Build history of the part. All positions in model axes, mm. A direction names the side the tool comes from. Give positions to 0.01 mm unless a question says otherwise; leave off trailing zeros. Order: outer loops, then holes, each group sorted by start corner. A loop starts at its lowest first (then second) coordinate and runs counter-clockwise, first axis right, second up. Notation, with made-up numbers: (8.5, -14.75) - (49.5, -14.75) arc R25 cw to (49.5, 7.25) - close; hole circle Ø9 at (60.25, -11.75). An arc over 180 degrees is marked (long way). Answer in a Markdown table with one row per item.
```python
from build123d import *

# Parameters (mm, degrees)
SKETCH1_R           = 9.5
BOSS_EXTRUDE1_DEPTH = 35
EXTRUDE_THIN1_START = 0.5
SKETCH1_4_R         = 5.5
SKETCH1_4_R_2       = 5
EXTRUDE_THIN1_DEPTH = 28.5
BOSS_EXTRUDE2_START = 0.8
SKETCH1_5_R         = 8.5
SKETCH1_5_R_2       = 5
BOSS_EXTRUDE2_DEPTH = 28
BOSS_EXTRUDE3_START = 0.3
SKETCH1_6_R         = 9.5
SKETCH1_6_R_2       = 8.5
BOSS_EXTRUDE3_DEPTH = 30
BOSS_EXTRUDE4_START = 1
BOSS_EXTRUDE4_DEPTH = 1
FILLET1_R           = 0.5
SKETCH4_R           = 2.15
CUT_EXTRUDE3_DEPTH  = 48.968739894
CHAMFER1_SIZE       = 1


with BuildPart() as part:
    # Sketch1 → Boss-Extrude1 (new body)
    with BuildSketch(Plane(origin=(0, 0, 0), x_dir=(0, 0, -1), z_dir=(1, 0, 0))):
        Polygon((-20, -5), (-18.5, -3.5), (-18.5, 8), (-9.5, 8), (-5, 13), (5, 13), (9.5, 8), (18.5, 8), (18.5, -3.5), (20, -5), (20, -13), (10, -13), (8.5, -11.5), (-8.5, -11.5), (-10, -13), (-20, -13), align=None)
        Circle(SKETCH1_R, mode=Mode.SUBTRACT)
    extrude(amount=BOSS_EXTRUDE1_DEPTH)



with BuildPart() as body_2:
    # Sketch1_4 → Extrude-Thin1 (new body)
    with BuildSketch(Plane(origin=(0, 0, 0), x_dir=(0, 0, -1), z_dir=(1, 0, 0)).offset(EXTRUDE_THIN1_START)):
        Circle(SKETCH1_4_R)
        Circle(SKETCH1_4_R_2, mode=Mode.SUBTRACT)
    extrude(amount=EXTRUDE_THIN1_DEPTH)

    # Sketch1_5 → Boss-Extrude2 (add)
    with BuildSketch(Plane(origin=(0, 0, 0), x_dir=(0, 0, -1), z_dir=(1, 0, 0)).offset(BOSS_EXTRUDE2_START)):
        Circle(SKETCH1_5_R)
        with Locations(Location((0, 0, 0), (0, 0, 180))):
            Circle(SKETCH1_5_R_2, mode=Mode.SUBTRACT)
    extrude(amount=BOSS_EXTRUDE2_DEPTH)


with BuildPart() as part_1:
    add(part.part)

    add(body_2.part)  # Boss-Extrude3 merges body 2
    # Sketch1_6 → Boss-Extrude3 (add)
    with BuildSketch(Plane(origin=(0, 0, 0), x_dir=(0, 0, -1), z_dir=(1, 0, 0)).offset(BOSS_EXTRUDE3_START)):
        Circle(SKETCH1_6_R)
        Circle(SKETCH1_6_R_2, mode=Mode.SUBTRACT)
    extrude(amount=BOSS_EXTRUDE3_DEPTH)

    # Sketch3 → Boss-Extrude4 (add)
    with BuildSketch(Plane(origin=(30.3, 0, 0), x_dir=(0, 0, -1), z_dir=(1, 0, 0)).offset(BOSS_EXTRUDE4_START)):
        with BuildLine():
            Line((-1.015917942, -8.43907049), (-1.1354377, -9.431902312))
            ThreePointArc((-1.1354377, -9.431902312), (0, 9.5), (1.1354377, -9.431902312))
            Line((1.1354377, -9.431902312), (1.015917942, -8.43907049))
            ThreePointArc((1.015917942, -8.43907049), (1.500925976, -7.394796464), (2.647576922, -7.499355735))
            ThreePointArc((2.647576922, -7.499355735), (4.216931478, -7.125074609), (3.386935643, -5.741576507))
            ThreePointArc((3.386935643, -5.741576507), (0, 6.666110848), (-3.386935643, -5.741576507))
            ThreePointArc((-3.386935643, -5.741576507), (-4.216931478, -7.125074609), (-2.647576922, -7.499355735))
            ThreePointArc((-2.647576922, -7.499355735), (-1.500925976, -7.394796464), (-1.015917942, -8.43907049))
        make_face()
    extrude(amount=BOSS_EXTRUDE4_DEPTH)

    # Fillet1
    fillet1_edges = [part_1.edges().sort_by_distance(p)[0] for p in [
        (35, -4.25, 19.25),
        (35, -9, 20),
        (0, 2.25, 18.5),
        (0, 8, 14),
        (0, 10.5, 7.25),
        (0, 13, 0),
        (0, 10.5, -7.25),
        (0, 8, -14),
        (0, 2.25, -18.5),
        (0, -4.25, -19.25),
        (0, -9, -20),
        (0, -9, 20),
        (0, -4.25, 19.25),
        (17.5, -3.5, 18.5),
        (17.5, 8, 18.5),
        (17.5, 8, 9.5),
        (17.5, 13, 5),
        (17.5, 13, -5),
        (17.5, 8, -9.5),
        (17.5, 8, -18.5),
        (17.5, -3.5, -18.5),
        (17.5, -5, -20),
        (17.5, -5, 20),
        (35, -9, -20),
        (35, -4.25, -19.25),
        (35, 2.25, -18.5),
        (35, 8, -14),
        (35, 10.5, -7.25),
        (35, 13, 0),
        (35, 10.5, 7.25),
        (35, 8, 14),
        (35, 2.25, 18.5),
    ]]
    fillet(fillet1_edges, radius=FILLET1_R)

    # Sketch4 → Cut-Extrude3 (cut, through all)
    with BuildSketch(Plane.XZ.offset(13)):
        with Locations(Location((7, 14, 0), (0, 0, 270))):
            Circle(SKETCH4_R)
        with Locations(Location((28, 14, 0), (0, 0, 270))):
            Circle(SKETCH4_R)
        with Locations(Location((28, -14, 0), (0, 0, 270))):
            Circle(SKETCH4_R)
        with Locations(Location((7, -14, 0), (0, 0, 270))):
            Circle(SKETCH4_R)
    extrude(amount=-CUT_EXTRUDE3_DEPTH, mode=Mode.SUBTRACT)

    # Chamfer1
    chamfer1_edges = [part_1.edges().sort_by_distance(p)[0] for p in [
        (7, 8, -11.85),
        (28, 8, -11.85),
        (28, 8, 16.15),
        (28, -13, 16.15),
        (7, 8, 16.15),
        (7, -13, 16.15),
    ]]
    chamfer(chamfer1_edges, length=CHAMFER1_SIZE)


solid = part_1.part
```
1. Drop flat-ended pins along their axis: P1, Ø2, axis at x = 20, z = 15.5, coming from the +Y side; P2, Ø9.5, axis at y = 2.5, z = -1.5, coming from the +X side; P3, Ø4, axis at x = 7, z = 13, coming from the +Y side. Give the stop position or say it passes through.
Check result:
| item | result |
|---|---|
| P1 | stops at y = 8 |
| P2 | stops at x = 32.3 |
| P3 | stops at y = 7.85 |
2. Cut at A-A on z = -14. Write the cut outline in (x, y).
Check result:
| item | result |
|---|---|
| outline | (0, -13) - (4.85, -13) - (4.85, 7) - (3.85, 8) - (0.5, 8) arc R0.5 ccw to (0, 7.5) - close; (9.15, -13) - (25.85, -13) - (25.85, 7) - (24.85, 8) - (10.15, 8) - (9.15, 7) - close; (30.15, -13) - (35, -13) - (35, 7.5) arc R0.5 ccw to (34.5, 8) - (31.15, 8) - (30.15, 7) - close |
3. Two-plate mould, pull along X, no slides. Class faces 1 (the face through (17, -12, 9)), 2 (the face through (8.81, -2.63, 12.84)), 3 (the face through (0.15, -4.34, 19.14)), 4 (the face through (32.3, 2.3, -6.5)): +X half, -X half, draft (parallel to the pull), parting line (faces both ways), or undercut.
Check result:
| item | result |
|---|---|
| face 1 | draft |
| face 2 | undercut |
| face 3 | -X half |
| face 4 | +X half |
4. Cut at C-C on y = 0. Count the separate pieces of the cut face and the enclosed holes in it, and give its area (3 significant figures).
Check result:
| item | result |
|---|---|
| separate pieces | 2 |
| enclosed holes | 4 |
| area | 834 mm² |
5. Cut at D-D on z = 14. Write the cut outline in (x, y).
Check result:
| item | result |
|---|---|
| outline | (0, -13) - (3.85, -13) - (4.85, -12) - (4.85, 7) - (3.85, 8) - (0.5, 8) arc R0.5 ccw to (0, 7.5) - close; (9.15, -12) - (10.15, -13) - (24.85, -13) - (25.85, -12) - (25.85, 7) - (24.85, 8) - (10.15, 8) - (9.15, 7) - close; (30.15, -12) - (31.15, -13) - (35, -13) - (35, 7.5) arc R0.5 ccw to (34.5, 8) - (31.15, 8) - (30.15, 7) - close |
6. Cut at B-B on x = 22.5. Write the cut outline in (y, z).
Check result:
| item | result |
|---|---|
| outline | (-13, -20) - (-5.21, -20) arc R0.5 ccw to (-4.85, -19.85) - (-3.65, -18.65) arc R0.5 cw to (-3.29, -18.5) - (7.5, -18.5) arc R0.5 ccw to (8, -18) - (8, -9.72) arc R0.5 cw to (8.17, -9.35) - (12.83, -5.15) arc R0.5 ccw to (13, -4.78) - (13, 4.78) arc R0.5 ccw to (12.83, 5.15) - (8.17, 9.35) arc R0.5 cw to (8, 9.72) - (8, 18) arc R0.5 ccw to (7.5, 18.5) - (-3.29, 18.5) arc R0.5 cw to (-3.65, 18.65) - (-4.85, 19.85) arc R0.5 ccw to (-5.21, 20) - (-13, 20) - (-13, 10) - (-11.5, 8.5) - (-11.5, -8.5) - (-13, -10) - close; hole circle Ø10 at (0, 0) |
7. Which spindle directions (+Z, -Z, +X, -X, +Y, -Y) get a long thin tool onto all of the face, cutting with end or side? Do faces 5 (the face through (31.79, 6.66, -0.24)), 6 (the face through (17, 2, -18.5)), 7 (the face through (17, 13, 0)), 8 (the face through (0.15, -4.36, -19.16)), 9 (the face through (0.3, -8.4, 2.2)). Say none if no direction does.
Check result:
| item | result |
|---|---|
| face 5 | +X |
| face 6 | -Z, +X, -X, +Y |
| face 7 | +Z, -Z, +X, -X, +Y |
| face 8 | -Z, -X, +Y |
| face 9 | -X |
8. Probe line 1 (X direction, y = -7.5, z = 14); line 2 (X direction, y = 8, z = -2.5); line 3 (Y direction, x = 31, z = 0). List the from-to ranges inside material, lowest first.
Check result:
| item | result |
|---|---|
| line 1 | x = 0 to 4.85, 9.15 to 25.85, 30.15 to 35 |
| line 2 | x = 0.8 to 28.8, 31.3 to 32.3 |
| line 3 | y = -11.5 to -9.5, 9.5 to 13 |
